```python
from build123d import *

# Parameters (mm, degrees)
ESQUISSE1_W             = 190
ESQUISSE1_H             = 12
BOSS_EXTRU_1_DEPTH      = 2.5
BOSS_EXTRU_3_DEPTH      = 5.1
ENL_V_START             = -40
ESQUISSE5_W             = 12
ESQUISSE5_H             = 10.1
ENL_V_MAT_EXTRU_1_DEPTH = 151
CONG_1_R                = 0.5


with BuildPart() as part:
    # Esquisse1 → Boss.-Extru.1 (new body, symmetric)
    with BuildSketch(Plane(origin=(0, 0, 0), x_dir=(1, 0, 0), z_dir=(0, 1, 0))):
        Rectangle(ESQUISSE1_W, ESQUISSE1_H)
        with BuildLine():
            Line((-88, 2.5), (88, 2.5))
            ThreePointArc((88, 2.5), (90.5, 0), (88, -2.5))
            Line((88, -2.5), (-88, -2.5))
            ThreePointArc((-88, -2.5), (-90.5, 0), (-88, 2.5))
        make_face(mode=Mode.SUBTRACT)
    extrude(amount=BOSS_EXTRU_1_DEPTH, both=True)

    # Esquisse4 → Boss.-Extru.3 (add)
    with BuildSketch(Plane.XZ.offset(2.5)):
        with BuildLine():
            Line((-95, 6), (-75, 6))
            Line((-75, 6), (-75, 2.5))
            Line((-75, 2.5), (-88, 2.5))
            ThreePointArc((-88, 2.5), (-90.5, 0), (-88, -2.5))
            Line((-88, -2.5), (-75, -2.5))
            Line((-75, -2.5), (-75, -6))
            Line((-75, -6), (-95, -6))
            Line((-95, -6), (-95, 6))
        make_face()
    boss_extru_3 = extrude(amount=BOSS_EXTRU_3_DEPTH)

    # Symétrie2: Boss.-Extru.3 across plane
    add(boss_extru_3.mirror(Plane(origin=(0, 0, 0), x_dir=(0, 0, 1), z_dir=(1, 0, 0))))

    # Esquisse5 → Enlèv. mat.-Extru.1 (cut, through all)
    with BuildSketch(Plane.ZY.offset(95).offset(ENL_V_START)):
        with Locations((0, -2.55)):
            Rectangle(ESQUISSE5_W, ESQUISSE5_H)
    extrude(amount=-ENL_V_MAT_EXTRU_1_DEPTH, mode=Mode.SUBTRACT)

    # Congé1
    cong_1_edges = [part.edges().sort_by_distance(p)[0] for p in [
        (-95, 2.5, 0),
        (-90.5, 2.5, 0),
        (-75, 2.5, 6),
        (-71.5, 2.5, 2.5),
        (-65, -2.5, 6),
        (-65, -2.5, 2.5),
        (-75, -2.5, -4.25),
        (-75, -5.05, -6),
        (-75, -5.05, -2.5),
        (-75, -2.5, 4.25),
        (-75, -5.05, 2.5),
        (-75, -5.05, 6),
        (-95, -7.6, 0),
        (-85, -7.6, -6),
        (-75, -7.6, -4.25),
        (-81.5, -7.6, -2.5),
        (-90.5, -7.6, 0),
        (-81.5, -7.6, 2.5),
        (-75, -7.6, 4.25),
        (-85, -7.6, 6),
        (-65, -2.5, -2.5),
        (-71.5, 2.5, -2.5),
        (-55, 0, -2.5),
        (-65, -2.5, -6),
        (-95, -2.55, 6),
        (-75, 2.5, -6),
        (-95, -2.55, -6),
        (-55, -2.5, 4.25),
        (-55, 0, 2.5),
        (-55, -2.5, -4.25),
        (-55, 0, 6),
        (-55, 2.5, 4.25),
        (-55, 2.5, -4.25),
        (-55, 0, -6),
    ]]
    fillet(cong_1_edges, radius=CONG_1_R)


solid = part.part
```
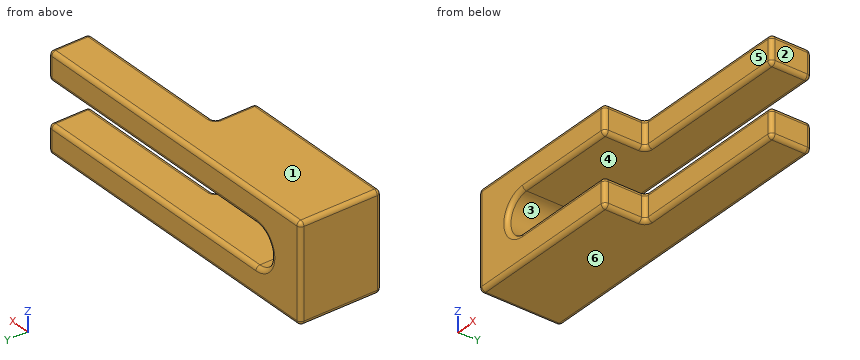
Check sheet for the modelled part. Datum: model origin and axes. Units: mm. Face numbers are marked on the shaded views. A direction names the side the tool comes from. Give positions to 0.01 mm unless a question says otherwise; leave off trailing zeros. Order: outer loops, then holes, each group sorted by start corner. A loop starts at its lowest first (then second) coordinate and runs counter-clockwise, first axis right, second up. Notation, with made-up numbers: (70, 35.5) -> (109, 35.5) arc R24 ccw to (109, 46.5) -> close; hole circle Ø5 at (13.5, 18.25). An arc over 180 degrees is marked (long way). Use CSV: the item, a comma, the result in double quotes. Start each with the question number.
1) Sectioned sample at C-C, the plane z = -3.5. Record the boundary of the cut face in (x, y).
2) Sectioned sample at B-B, the plane y = -4.75. Record the boundary of the cut face in (x, z), plus the area to 3 significant figures.
3) Material ranges on line 1 (Z direction, x = -81.5, y = -6.75); line 2 (X direction, y = -4.75, z = 4.75); line 3 (Y direction, x = -70.5, z = -3.75), recorded low to high. Write a range as from..to.
4) Sectioned sample at D-D, the plane x = -85.5. Record the boundary of the cut face in (y, z).
5) Set-up check for the marked faces 4, 5 and 6: record each of +Z, -Z, +X, -X, +Y, -Y from which the full face is reachable in a straight line by a thin tool's end or side.
6) Go/stop test with flat-tipped pins: P1, Ø1.2, axis at x = -64, z = 4.5, coming from the -Y side; P2, Ø0.8, axis at y = -5, z = -4, coming from the +X side. Record where each tip stops, or that it passes through.
7) Sectioned sample at A-A, the plane x = -62. Record the boundary of the cut face in (y, z), plus the area to 3 significant figures.
8) Mould release check, pull along Z, two halves, no side actions. Record for the marked faces 1, 2 and 3: released by +Z, released by -Z, zero draft, split by the parting line, or undercut.
Recorded:
1,outline,"(-95, -7.1) arc R0.5 ccw to (-94.5, -7.6) -> (-75.5, -7.6) arc R0.5 ccw to (-75, -7.1) -> (-75, -3) arc R0.5 cw to (-74.5, -2.5) -> (-55.5, -2.5) arc R0.5 ccw to (-55, -2) -> (-55, 2) arc R0.5 ccw to (-55.5, 2.5) -> (-94.5, 2.5) arc R0.5 ccw to (-95, 2) -> close"
2,outline,"(-95, -5.5) arc R0.5 ccw to (-94.5, -6) -> (-75.5, -6) arc R0.5 ccw to (-75, -5.5) -> (-75, -3) arc R0.5 ccw to (-75.5, -2.5) -> (-88, -2.5) arc R2.5 cw to (-88, 2.5) -> (-75.5, 2.5) arc R0.5 ccw to (-75, 3) -> (-75, 5.5) arc R0.5 ccw to (-75.5, 6) -> (-94.5, 6) arc R0.5 ccw to (-95, 5.5) -> close"
2,area,"165 mm2"
3,line 1,"-6..-2.5, 2.5..6"
3,line 2,"-95..-75"
3,line 3,"-2.5..2.5"
4,outline,"(-7.6, -5.5) arc R0.5 ccw to (-7.1, -6) -> (2, -6) arc R0.5 ccw to (2.5, -5.5) -> (2.5, -3) arc R0.5 ccw to (2, -2.5) -> (-7.1, -2.5) arc R0.5 ccw to (-7.6, -3) -> close; (-7.6, 3) arc R0.5 ccw to (-7.1, 2.5) -> (2, 2.5) arc R0.5 ccw to (2.5, 3) -> (2.5, 5.5) arc R0.5 ccw to (2, 6) -> (-7.1, 6) arc R0.5 ccw to (-7.6, 5.5) -> close"
5,face 4,"+X, +Y, -Y"
5,face 5,"+Z, -Z, +X, -Y"
5,face 6,"-Z, +X, -X, +Y, -Y"
6,P1,"y = -2.5"
6,P2,"x = -75"
7,outline,"(-2.5, -5.5) arc R0.5 ccw to (-2, -6) -> (2, -6) arc R0.5 ccw to (2.5, -5.5) -> (2.5, -3) arc R0.5 ccw to (2, -2.5) -> (-2, -2.5) arc R0.5 ccw to (-2.5, -3) -> close; (-2.5, 3) arc R0.5 ccw to (-2, 2.5) -> (2, 2.5) arc R0.5 ccw to (2.5, 3) -> (2.5, 5.5) arc R0.5 ccw to (2, 6) -> (-2, 6) arc R0.5 ccw to (-2.5, 5.5) -> close"
7,area,"34.6 mm2"
8,face 1,"released by +Z"
8,face 2,"zero draft"
8,face 3,"undercut"
